Geometry check sheet. Reference: drawing and pictorial views, mm from the part's lowest x, y, z. Give positions to 0.01 mm unless a question says otherwise; leave off trailing zeros. Order: outer loops, then holes, each group sorted by start corner. A loop starts at its lowest first (then second) coordinate and runs counter-clockwise, first axis right, second up.
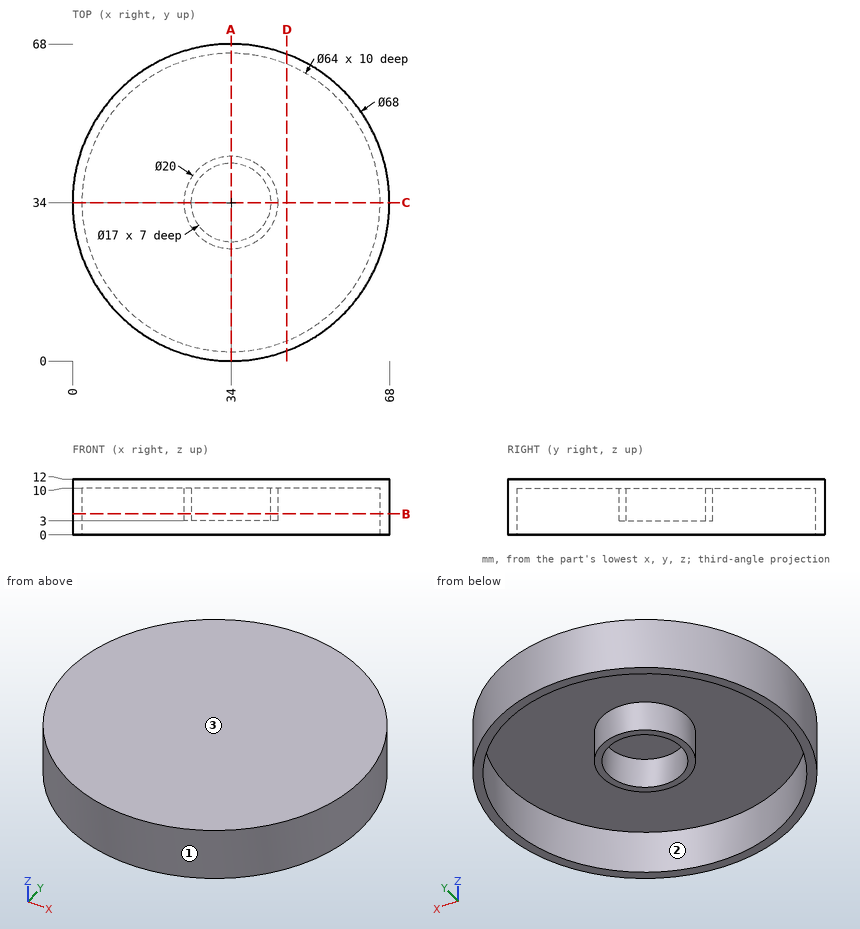
1) Depth check by flat-ended pin: pin 1 Ø1.5 at (y, z) = (26, 8) entering from -X; pin 2 Ø1.5 at (y, z) = (26, 7) entering from +X; pin 3 Ø6 at (x, z) = (33, 8) entering from +Y; pin 4 Ø1.5 at (x, y) = (61, 58.5) entering from +Z. Enter the tip coordinate at first touch or a pass-through.
Recorded:
pin 1: stops at x = 0.78
pin 2: stops at x = 67.22
pin 3: stops at y = 68
pin 4: passes through
2) Draft check along X on the marked faces 1, 2 and 3. Enter one of: +X half, -X half, draft (parallel to the pull), parting line (faces both ways), or undercut.
Recorded:
face 1: parting line
face 2: undercut
face 3: draft
3) Material ranges on L1, parallel to Y at x = 34, z = 5; L2, parallel to X at y = 31.5, z = 3.5; L3, parallel to Z at x = 37, y = 38, recorded low to high.
Recorded:
L1: y = 0 to 2, 24 to 25.5, 42.5 to 44, 66 to 68
L2: x = 0.09 to 2.1, 24.32 to 25.88, 42.12 to 43.68, 65.9 to 67.91
L3: z = 10 to 12
4) Section check A-A, the plane x = 34. Record the cut outline in (y, z).
Recorded:
outline: (0, 0) - (2, 0) - (2, 10) - (24, 10) - (24, 3) - (25.5, 3) - (25.5, 10) - (42.5, 10) - (42.5, 3) - (44, 3) - (44, 10) - (66, 10) - (66, 0) - (68, 0) - (68, 12) - (0, 12) - close
5) Section check B-B, the plane z = 4.5. Record the cut outline in (x, y).
Recorded:
outline: circle Ø68 at (34, 34); circle Ø20 at (34, 34); hole circle Ø64 at (34, 34); hole circle Ø17 at (34, 34)
6) Section check D-D, the plane x = 46. Record the cut outline in (y, z).
Recorded:
outline: (2.19, 0) - (4.34, 0) - (4.34, 10) - (63.66, 10) - (63.66, 0) - (65.81, 0) - (65.81, 12) - (2.19, 12) - close
